from build123d import *

# Parameters (mm, degrees)
SKETCH2_R          = 2.5
CUT_EXTRUDE1_DEPTH = 56
SKETCH3_R          = 1.75
CUT_EXTRUDE2_DEPTH = 10


with BuildPart() as part:
    # Sketch1 → Revolve1 (revolve)
    with BuildSketch(Plane.XY, mode=Mode.PRIVATE) as revolve1_sk:
        Polygon((0, 16.8), (2, 16.8), (2, 14), (11.75, 14), (11.75, 12.75), (6.2, 12.75), (6.2, 0), (0, 0), align=None)
    revolve(revolve1_sk.sketch.rotate(Axis((0, 0, 0), (0, 1, 0)), 90), axis=Axis((0, 0, 0), (0, 1, 0)))

    # Sketch2 → Cut-Extrude1 (cut)
    with BuildSketch(Plane(origin=(0, 16.8, 0), x_dir=(1, 0, 0), z_dir=(0, 1, 0))):
        with Locations(Location((0, 0, 0), (0, 0, 270))):
            Circle(SKETCH2_R)
    extrude(amount=-CUT_EXTRUDE1_DEPTH, mode=Mode.SUBTRACT)

    # Sketch3 → Cut-Extrude2 (cut)
    with BuildSketch(Plane(origin=(0, 14, 0), x_dir=(1, 0, 0), z_dir=(0, 1, 0))):
        with Locations(Location((0, 9, 0), (0, 0, 270))):
            Circle(SKETCH3_R)
        with Locations(Location((7.794228634, -4.5, 0), (0, 0, 270))):
            Circle(SKETCH3_R)
        with Locations(Location((-7.794228634, -4.5, 0), (0, 0, 270))):
            Circle(SKETCH3_R)
    extrude(amount=-CUT_EXTRUDE2_DEPTH, mode=Mode.SUBTRACT)


solid = part.part
For this review, take the finished solid that the model builds, in its own axes (mm). A direction names the side the tool comes from. Give positions to 0.01 mm unless a question says otherwise; leave off trailing zeros. Loops run counter-clockwise (first coordinate to the right, second up) from the corner with the lowest first, then second, coordinate; pieces in that order, holes last. Notation, with made-up numbers: (35.25, 34) -> (91.25, 34) arc R18 cw to (91.25, 60) -> close; hole circle Ø4 at (6, 68). An arc over 180 degrees is marked (long way). One line per question, with ' | ' between items.
1) We need section C-C (x = -8.75). Write out the cut boundary in (y, z), plus the area to 3 significant figures.
Resolved:
outline: (12.75, -7.84) -> (14, -7.84) -> (14, 3.03) -> (12.75, 3.03) -> close; (12.75, 5.97) -> (14, 5.97) -> (14, 7.84) -> (12.75, 7.84) -> close | area: 15.9 mm2
2) The part is to be moulded in two halves that separate along Y. For faces 3 (the cylindrical face through (-11.65, 13.37, 1.53)), 4 (the flat face through (5, 12.75, -5)), 5 (the flat face through (-3, 14, 0)), say which applies: +Y half, -Y half, draft (parallel to the pull), parting line (faces both ways), or undercut.
Resolved:
face 3: draft | face 4: -Y half | face 5: +Y half
3) To check wall thickness, follow probe 1 along X at (y, z) = (3.25, 0); probe 2 along Z at (x, y) = (-1, 13.75); probe 3 along Y at (x, z) = (2, 9.75). State the ranges of each line that lie inside material, in increasing order.
Resolved:
probe 1: x = -6.2 to -2.5, 2.5 to 6.2 | probe 2: z = -11.71 to -10.44, -7.56 to -2.29, 2.29 to 11.71 | probe 3: y = 12.75 to 14
4) We need section D-D (z = 4.5). Write out the cut boundary in (x, y), plus the area to 3 significant figures.
Resolved:
outline: (-10.85, 12.75) -> (-9.54, 12.75) -> (-9.54, 14) -> (-10.85, 14) -> close; (-6.04, 12.75) -> (-4.26, 12.75) -> (-4.26, 0) -> (4.26, 0) -> (4.26, 12.75) -> (6.04, 12.75) -> (6.04, 14) -> (-6.04, 14) -> close; (9.54, 12.75) -> (10.85, 12.75) -> (10.85, 14) -> (9.54, 14) -> close | area: 127 mm2
5) We need section B-B (z = 0). Write out the cut boundary in (x, y), plus the area to 3 significant figures.
Resolved:
outline: (-11.75, 12.75) -> (-6.2, 12.75) -> (-6.2, 0) -> (-2.5, 0) -> (-2.5, 14) -> (-11.75, 14) -> close; (2.5, 0) -> (6.2, 0) -> (6.2, 12.75) -> (11.75, 12.75) -> (11.75, 14) -> (2.5, 14) -> close | area: 117 mm2
6) We need section A-A (x = 0). Write out the cut boundary in (y, z).
Resolved:
outline: (0, -6.2) -> (12.75, -6.2) -> (12.75, -7.25) -> (14, -7.25) -> (14, -2.5) -> (0, -2.5) -> close; (0, 2.5) -> (14, 2.5) -> (14, 11.75) -> (12.75, 11.75) -> (12.75, 6.2) -> (0, 6.2) -> close; (12.75, -11.75) -> (14, -11.75) -> (14, -10.75) -> (12.75, -10.75) -> close
7) For faces 1 (the cylindrical face through (-1.9, 6.3, -5.9)), 2 (the cylindrical face through (-7.72, 13.38, 2.75)), list the 3-axis set-ups (+Z, -Z, +X, -X, +Y, -Y) from which the entire face can be reached by the end or side of a thin tool; tool diameter is ignored.
Resolved:
face 1: -Y | face 2: +Y, -Y
8) Insertion check: pin 1 Ø4.5 at (x, z) = (7.79, 4.5) entering from -Y; pin 2 Ø2 at (x, z) = (-7.79, 4.5) entering from -Y; pin 3 Ø6 at (x, y) = (-1.5, 9.5) entering from -Z; pin 4 Ø6 at (y, z) = (7, -6) entering from -X. Each pin has a flat end and moves straight along its axis. Give the tip position at first contact, or say it passes through.
Resolved:
pin 1: stops at y = 12.75 | pin 2: passes through | pin 3: stops at z = -6.2 | pin 4: stops at x = -5.43
